Drawing for the job (mm, zero at the part's lowest x, y, z). A direction names the side the tool comes from. Round coordinates to 2 decimals unless told otherwise and drop trailing zeros. Write each loop counter-clockwise with the first axis right and the second up, starting at its lowest first coordinate (ties: lowest second). Pieces come first, ordered by that corner, then holes. Notation, with made-up numbers: M 61,65 L 66,65 A24 cw 66,87 Z; hole C 63,-5 d6. An arc over 180 degrees is marked long. Use a Markdown table: item, result.
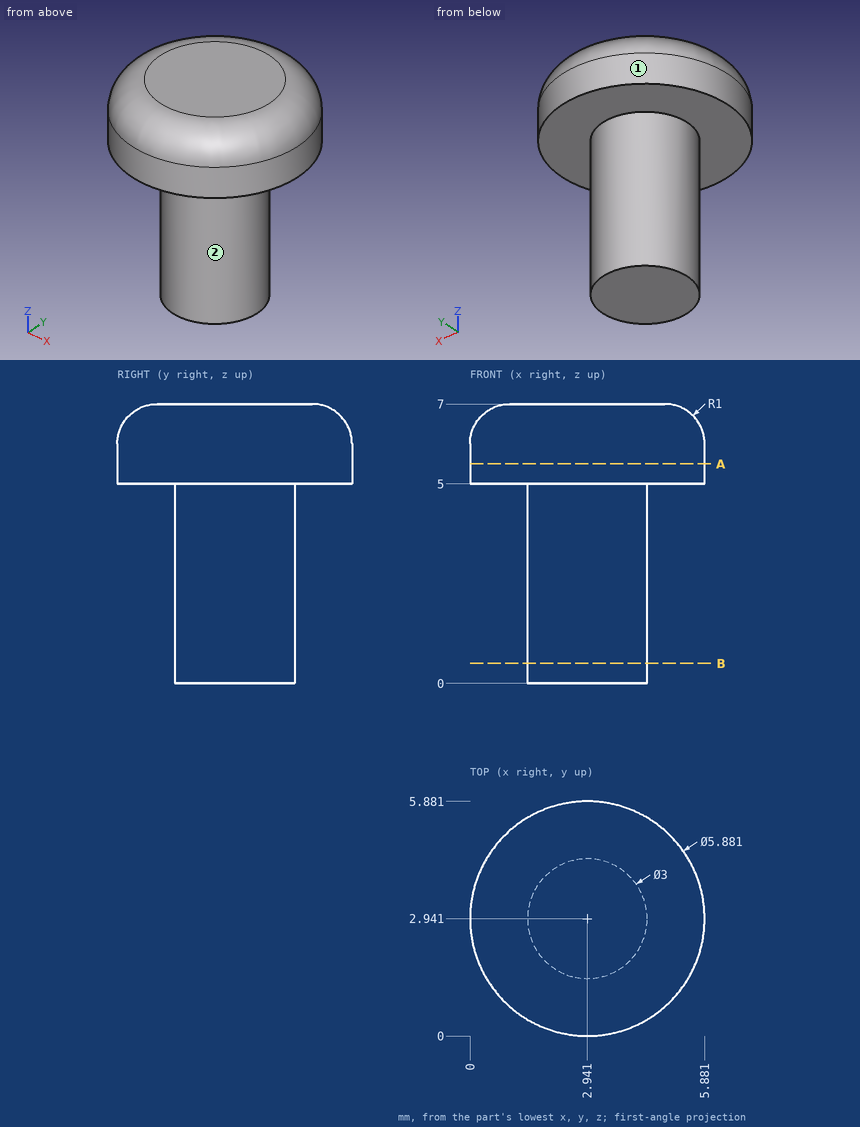
Q1. Drop flat-ended pins along their axis: P1, Ø2, axis at x = 3.5, z = 5.5, coming from the -Y side; P2, Ø2, axis at x = 4.5, z = 3.5, coming from the -Y side; P3, Ø2, axis at x = 5, z = 2, coming from the -Y side; P4, Ø2, axis at y = 2, z = 3, coming from the +X side. Give the stop position or say it passes through.
Response values:
| item | result |
|---|---|
| P1 | stops at y = 0 |
| P2 | stops at y = 1.55 |
| P3 | stops at y = 1.88 |
| P4 | stops at x = 4.44 |
Q2. Cut at B-B on z = 0.5. Give the cut face in (x, y).
Response values:
| item | result |
|---|---|
| outline | C 2.94,2.94 d3 |
Q3. Which spindle directions (+Z, -Z, +X, -X, +Y, -Y) get a long thin tool onto all of the face, cutting with end or side? Do the marked faces 1 and 2. Say none if no direction does.
Response values:
| item | result |
|---|---|
| face 1 | +Z, -Z |
| face 2 | -Z |
Q4. Cut at A-A on z = 5.5. Give the cut face in (x, y), and give its area (3 significant figures).
Response values:
| item | result |
|---|---|
| outline | C 2.94,2.94 d5.88 |
| area | 27.2 mm2 |
Q5. Drill centre lines: L1, parallel to Z at x = 4.55, y = 2.35; L2, parallel to X at y = 3.6, z = 1.5; L3, parallel to Y at x = 4.1, z = 6.75. Where is each one in solid material? Low to high.
Response values:
| item | result |
|---|---|
| L1 | z = 5 to 7 |
| L2 | x = 1.59 to 4.29 |
| L3 | y = 0.61 to 5.27 |
